from build123d import *

# Parameters (mm, degrees)
BOSS_EXTRUDE1_DEPTH = 13
SKETCH2_R           = 1.65
CUT_EXTRUDE1_DEPTH  = 22.90006621
FILLET2_R           = 4


with BuildPart() as part:
    # Sketch1 → Boss-Extrude1 (new body)
    with BuildSketch(Plane.XY):
        with BuildLine():
            Line((-13.77, 5.5), (-13.77, -5.5))
            Line((-13.77, -5.5), (13.77, -5.5))
            Line((13.77, -5.5), (13.77, 5.5))
            Line((13.77, 5.5), (7.533923281, 5.5))
            ThreePointArc((7.533923281, 5.5), (0, -1.1), (-7.533923281, 5.5))
            Line((-7.533923281, 5.5), (-13.77, 5.5))
        make_face()
    extrude(amount=BOSS_EXTRUDE1_DEPTH)

    # Sketch2 → Cut-Extrude1 (cut, through all)
    with BuildSketch(Plane(origin=(0, 5.5, 0), x_dir=(1, 0, 0), z_dir=(0, 1, 0))):
        with Locations(Location((-10.65196164, -6.5, 0), (0, 0, 270))):
            Circle(SKETCH2_R)
        with Locations(Location((10.65196164, -6.5, 0), (0, 0, 270))):
            Circle(SKETCH2_R)
    extrude(amount=-CUT_EXTRUDE1_DEPTH, mode=Mode.SUBTRACT)

    # Fillet2
    fillet2_edges = [part.edges().sort_by_distance(p)[0] for p in [
        (-13.77, 0, 13),
        (13.77, 0, 13),
        (13.77, 0, 0),
        (-13.77, 0, 0),
    ]]
    fillet(fillet2_edges, radius=FILLET2_R)


solid = part.part
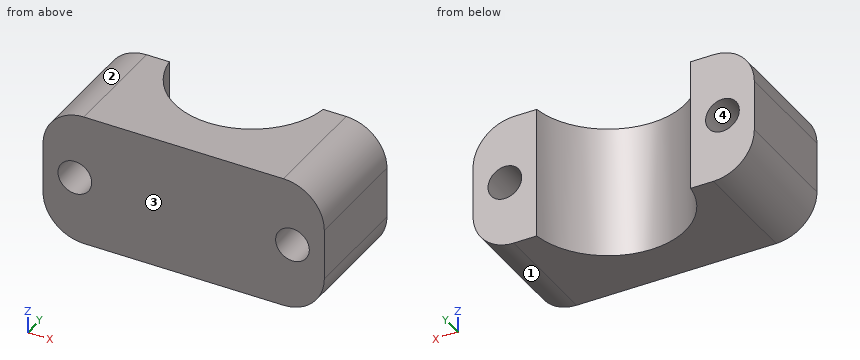
Could you check a few things on this model? Use its own coordinates, in mm. Face numbers are marked on the shaded views. Give positions to 0.01 mm unless a question says otherwise; leave off trailing zeros. Order: outer loops, then holes, each group sorted by start corner. A loop starts at its lowest first (then second) coordinate and runs counter-clockwise, first axis right, second up. Notation, with made-up numbers: (-18.5, -26.5) -> (14.5, -26.5) arc R28 ccw to (14.5, 12.5) -> close; hole circle Ø8 at (57, 51). An arc over 180 degrees is marked (long way). Return JSON: item names as keys, results as strings.
1. Imagine slicing it at D-D on z = 1.5. List the corners of the cut face in (x, y) for me.
Answer list:
{"outline": "(-12.89, -5.5) -> (12.89, -5.5) -> (12.89, 5.5) -> (7.53, 5.5) arc R7.6 cw to (-7.53, 5.5) -> (-12.89, 5.5) -> close"}
2. For pin 1 Ø5 at (x, y) = (-5.5, 3) entering from +Z; pin 2 Ø2.5 at (x, z) = (-10.65, 6.5) entering from -Y; pin 3 Ø2 at (y, z) = (1.5, 2) entering from +X; pin 4 Ø2 at (x, z) = (-0.5, 1.5) entering from +Y, each with a flat end and sliding along its axis, tell me the tip position at first contact or that it passes through.
Answer list:
{"pin 1": "stops at z = 13", "pin 2": "passes through", "pin 3": "stops at x = 13.64", "pin 4": "stops at y = -0.95"}
3. Thinking about a two-plate mould opening in Z: for the marked faces 1, 2, 3 and 4, which applies, pulls with the +Z half, pulls with the -Z half, needs draft (parallel to the pull), parting line crosses it, or undercut?
Answer list:
{"face 1": "pulls with the -Z half", "face 2": "pulls with the +Z half", "face 3": "needs draft", "face 4": "undercut"}
4. Imagine slicing it at C-C on y = -2. List the corners of the cut face in (x, z) for me, then the cut area to 3 significant figures.
Answer list:
{"outline": "(-13.77, 4) arc R4 ccw to (-9.77, 0) -> (9.77, 0) arc R4 ccw to (13.77, 4) -> (13.77, 9) arc R4 ccw to (9.77, 13) -> (-9.77, 13) arc R4 ccw to (-13.77, 9) -> close; hole circle Ø3.3 at (-10.65, 6.5); hole circle Ø3.3 at (10.65, 6.5)", "area": "327 mm2"}
5. I need wall thicknesses on line 1 (X direction, y = -1.25, z = 6.5); line 2 (X direction, y = 2.5, z = 6.5); line 3 (X direction, y = 0, z = 6.5). Which ranges of each line are inside material? Lowest first, please. Write a range as from..to.
Answer list:
{"line 1": "x = -13.77..-12.3, -9..9, 12.3..13.77", "line 2": "x = -13.77..-12.3, -9..-6.46, 6.46..9, 12.3..13.77", "line 3": "x = -13.77..-12.3, -9..-3.94, 3.94..9, 12.3..13.77"}
6. Imagine slicing it at B-B on y = 2.5. List the corners of the cut face in (x, z) for me.
Answer list:
{"outline": "(-13.77, 4) arc R4 ccw to (-9.77, 0) -> (-6.46, 0) -> (-6.46, 13) -> (-9.77, 13) arc R4 ccw to (-13.77, 9) -> close; (6.46, 0) -> (9.77, 0) arc R4 ccw to (13.77, 4) -> (13.77, 9) arc R4 ccw to (9.77, 13) -> (6.46, 13) -> close; hole circle Ø3.3 at (-10.65, 6.5); hole circle Ø3.3 at (10.65, 6.5)"}
7. Imagine slicing it at A-A on z = 6.5. List the corners of the cut face in (x, y) for me, then the cut area to 3 significant figures.
Answer list:
{"outline": "(-13.77, -5.5) -> (-12.3, -5.5) -> (-12.3, 5.5) -> (-13.77, 5.5) -> close; (-9, -5.5) -> (9, -5.5) -> (9, 5.5) -> (7.53, 5.5) arc R7.6 cw to (-7.53, 5.5) -> (-9, 5.5) -> close; (12.3, -5.5) -> (13.77, -5.5) -> (13.77, 5.5) -> (12.3, 5.5) -> close", "area": "155 mm2"}
